from build123d import *

# Parameters (mm, degrees)
F1_DEPTH       = 4
F2_W           = 29
F2_H           = 25
F3_DEPTH       = 2
F4_W           = 24
F4_H           = 21
F5_DEPTH       = 2
F7_D           = 3
F7_CSINK_D     = 6
F7_CSINK_ANGLE = 90
F8_D           = 3
F8_CSINK_D     = 6
F8_CSINK_ANGLE = 90


with BuildPart() as f1:
    # F0 (on Top) → F1 (new body)
    with BuildSketch(Plane.XY):
        with BuildLine():
            Line((-16.5, -17.5), (16.5, -17.5))
            ThreePointArc((16.5, -17.5), (20.035534, -16.035534), (21.5, -12.5))
            Line((21.5, -12.5), (21.5, 12.5))
            ThreePointArc((21.5, 12.5), (20.035534, 16.035534), (16.5, 17.5))
            Line((16.5, 17.5), (-16.5, 17.5))
            ThreePointArc((-16.5, 17.5), (-20.035534, 16.035534), (-21.5, 12.5))
            Line((-21.5, 12.5), (-21.5, -12.5))
            ThreePointArc((-21.5, -12.5), (-20.035534, -16.035534), (-16.5, -17.5))
        make_face()
    extrude(amount=F1_DEPTH)

    # F2 (on face) → F3 (cut)
    with BuildSketch(Plane.XY.offset(4)):
        Rectangle(F2_W, F2_H)
    extrude(amount=-F3_DEPTH, mode=Mode.SUBTRACT)

    # F4 (on face) → F5 (cut)
    with BuildSketch(Plane.XY.offset(2)):
        Rectangle(F4_W, F4_H)
    extrude(amount=-F5_DEPTH, mode=Mode.SUBTRACT)

    # F7 (through all)
    with Locations(Plane.XY.offset(4)):
        with Locations((-18, 0)):
            CounterSinkHole(F7_D / 2, F7_CSINK_D / 2, counter_sink_angle=F7_CSINK_ANGLE)

    # F8 (through all)
    with Locations(Plane.XY.offset(4)):
        with Locations((18, 0)):
            CounterSinkHole(F8_D / 2, F8_CSINK_D / 2, counter_sink_angle=F8_CSINK_ANGLE)


solid = f1.part
Check sheet for the modelled part. Datum: model origin and axes. Units: mm. A direction names the side the tool comes from. Coordinates: 2 decimals unless noted, no trailing zeros. Write each loop counter-clockwise with the first axis right and the second up, starting at its lowest first coordinate (ties: lowest second). Pieces come first, ordered by that corner, then holes.
Item 1: Access from +Z, -Z, +X, -X, +Y, -Y to the whole of each face (thin tool, end or side, straight path). Record for faces 4 (the face through (-14.5, 0, 3)), 5 (the face through (-21.5, 0, 2)), 6 (the face through (-12, 0, 1)).
Numbers:
face 4: +Z
face 5: +Z, -Z, -X, +Y, -Y
face 6: +Z, -Z
Item 2: Cross-section at B-B on y = 0. Record the boundary of the cut face in (x, z).
Numbers:
outline: (-21.5, 0) - (-19.5, 0) - (-19.5, 2.5) - (-21, 4) - (-21.5, 4) - close; (-16.5, 0) - (-12, 0) - (-12, 2) - (-14.5, 2) - (-14.5, 4) - (-15, 4) - (-16.5, 2.5) - close; (12, 0) - (16.5, 0) - (16.5, 2.5) - (15, 4) - (14.5, 4) - (14.5, 2) - (12, 2) - close; (19.5, 0) - (21.5, 0) - (21.5, 4) - (21, 4) - (19.5, 2.5) - close
Item 3: Scan lines: probe 1 along X at (y, z) = (0, 0.95); probe 2 along Y at (x, z) = (-3, 3.65); probe 3 along X at (y, z) = (-6, 0.3). Record each from-to range of solid material in increasing order.
Numbers:
probe 1: x = -21.5 to -19.5, -16.5 to -12, 12 to 16.5, 19.5 to 21.5
probe 2: y = -17.5 to -12.5, 12.5 to 17.5
probe 3: x = -21.5 to -12, 12 to 21.5
Item 4: Cross-section at C-C on z = 0.9. Record the boundary of the cut face in (x, y).
Numbers:
outline: (-21.5, -12.5) arc R5 ccw to (-16.5, -17.5) - (16.5, -17.5) arc R5 ccw to (21.5, -12.5) - (21.5, 12.5) arc R5 ccw to (16.5, 17.5) - (-16.5, 17.5) arc R5 ccw to (-21.5, 12.5) - close; hole circle Ø3 at (-18, 0); hole (-12, -10.5) - (12, -10.5) - (12, 10.5) - (-12, 10.5) - close; hole circle Ø3 at (18, 0)
Item 5: Cross-section at A-A on x = -10.5. Record the boundary of the cut face in (y, z), then the cut area to 3 significant figures.
Numbers:
outline: (-17.5, 0) - (-10.5, 0) - (-10.5, 2) - (-12.5, 2) - (-12.5, 4) - (-17.5, 4) - close; (10.5, 0) - (17.5, 0) - (17.5, 4) - (12.5, 4) - (12.5, 2) - (10.5, 2) - close
area: 48.0 mm2
Item 6: Mould release check, pull along X, two halves, no side actions. Record for faces 1 (the face through (12, 0, 1)), 2 (the face through (0, 12, 0)), 3 (the face through (-20.07, -16, 1.97)): released by +X, released by -X, zero draft, split by the parting line, or undercut.
Numbers:
face 1: undercut
face 2: zero draft
face 3: released by -X
Item 7: Cross-section at D-D on x = 12.5. Record the boundary of the cut face in (y, z).
Numbers:
outline: (-17.5, 0) - (17.5, 0) - (17.5, 4) - (12.5, 4) - (12.5, 2) - (-12.5, 2) - (-12.5, 4) - (-17.5, 4) - close
Item 8: Depth check by flat-ended pin: pin 1 Ø1.8 at (x, y) = (-18, 0) entering from -Z (3 decimals); pin 2 Ø20 at (x, y) = (3, 1) entering from +Z. Enter the tip coordinate at first touch or a pass-through.
Numbers:
pin 1: passes through
pin 2: stops at z = 2
